```python
from build123d import *

# Parameters (mm, degrees)
BOSS_EXTRU_2_DEPTH      = 151.845
BOSS_EXTRU_2_DEPTH_BACK = 151.845
ESQUISSE1_R             = 7
ESQUISSE3_W             = 68
ESQUISSE3_H             = 30
ESQUISSE3_H_2           = 35
ESQUISSE4_R             = 5
BOSS_EXTRU_3_DEPTH      = 15
BOSS_EXTRU_4_START      = 15
ESQUISSE5_R             = 5
BOSS_EXTRU_4_DEPTH      = 15
BOSS_EXTRU_6_DEPTH      = 2.5
BOSS_EXTRU_6_DEPTH_BACK = 2.5
ENL_V_START             = -68
ESQUISSE11_R            = 35
ESQUISSE11_R_2          = 30
ENL_V_MAT_EXTRU_1_DEPTH = 68


with BuildPart() as part:
    # Esquisse1 → Boss.-Extru.2 (new, two sides: drawn at the far end of the back side and taken through both)
    with BuildSketch(Plane(origin=(0, 0, 0), x_dir=(0, 0, -1), z_dir=(1, 0, 0)).offset(-BOSS_EXTRU_2_DEPTH_BACK)):
        Circle(ESQUISSE1_R)
    extrude(amount=BOSS_EXTRU_2_DEPTH + BOSS_EXTRU_2_DEPTH_BACK)

    # Esquisse3 → Révolution2 (revolve)
    with BuildSketch(Plane.XY, mode=Mode.PRIVATE) as r_volution2_sk:
        with Locations((-86.5, 15)):
            Rectangle(ESQUISSE3_W, ESQUISSE3_H)
        with Locations((86.5, 17.5)):
            Rectangle(ESQUISSE3_W, ESQUISSE3_H_2)
    revolve(r_volution2_sk.sketch.rotate(Axis((-120.5, 0, 0), (1, 0, 0)), 270), axis=Axis((-120.5, 0, 0), (1, 0, 0)))

    # Esquisse4 → Boss.-Extru.3 (add)
    with BuildSketch(Plane.ZY.offset(151.845)):
        Circle(ESQUISSE4_R)
    extrude(amount=BOSS_EXTRU_3_DEPTH)

    # Esquisse5 → Boss.-Extru.4 (add)
    with BuildSketch(Plane(origin=(151.845, 0, 0), x_dir=(0, 0, -1), z_dir=(1, 0, 0)).offset(BOSS_EXTRU_4_START)):
        with Locations(Location((0, 0, 0), (0, 0, 180))):
            Circle(ESQUISSE5_R)
    extrude(amount=-BOSS_EXTRU_4_DEPTH)

    # Esquisse6 → Boss.-Extru.6 (add, two sides: drawn at the far end of the back side and taken through both)
    with BuildSketch(Plane(origin=(0, 0, 0), x_dir=(0, 0, -1), z_dir=(1, 0, 0)).offset(-BOSS_EXTRU_6_DEPTH_BACK)):
        Polygon((-0.495363477, 14), (-2.169953885, 6.655170932), (-2.610793017, 6.495072622), (-8.616105681, 11.046145282), (-9.378598341, 10.406337972), (-5.940243898, 3.703466513), (-6.175037056, 3.29745816), (-13.700746567, 2.923641509), (-13.873589621, 1.94339984), (-6.931134583, -0.98116596), (-6.850019438, -1.443108535), (-12.374762678, -6.566901532), (-11.87708094, -7.428911588), (-4.678977177, -5.206734889), (-4.319908407, -5.508463622), (-5.258596613, -12.984753276), (-4.323260899, -13.325187635), (-0.237581159, -6.99604961), (0.231428968, -6.996382273), (4.31801844, -13.326929566), (5.253354154, -12.986495207), (4.314874913, -5.51186988), (4.674371346, -5.210650816), (11.874077864, -7.433322313), (12.371759603, -6.571312256), (6.848246248, -1.448659888), (6.93001661, -0.986832845), (13.87401748, 1.938384149), (13.701174426, 2.918625818), (6.177140243, 3.292359253), (5.942923274, 3.698700268), (9.382043313, 10.403064212), (8.619550653, 11.042871522), (2.615574856, 6.492811995), (2.174963279, 6.653535506), (0.5, 14), align=None)
    extrude(amount=BOSS_EXTRU_6_DEPTH + BOSS_EXTRU_6_DEPTH_BACK)

    # Esquisse11 → Enlèv. mat.-Extru.1 (cut)
    with BuildSketch(Plane(origin=(120.5, 0, 0), x_dir=(0, 0, -1), z_dir=(1, 0, 0)).offset(ENL_V_START)):
        Circle(ESQUISSE11_R)
        with Locations(Location((0, 0, 0), (0, 0, 180))):
            Circle(ESQUISSE11_R_2, mode=Mode.SUBTRACT)
    extrude(amount=ENL_V_MAT_EXTRU_1_DEPTH, mode=Mode.SUBTRACT)


solid = part.part
```
Could you check a few things on this model? Use its own coordinates, in mm. A direction names the side the tool comes from. Round coordinates to 2 decimals unless told otherwise and drop trailing zeros. Loops run counter-clockwise (first coordinate to the right, second up) from the corner with the lowest first, then second, coordinate; pieces in that order, holes last. Notation, with made-up numbers: (60, 50.5) -> (88, 50.5) arc R30 cw to (88, 87.5) -> close; hole circle Ø10 at (-23.5, 76). An arc over 180 degrees is marked (long way). Put each result on its own line as item: value.
Q1. I want a section at B-B on z = 22. Write out the boundary of the cut face in (x, y).
Checks:
outline: (-120.5, -20.4) -> (-52.5, -20.4) -> (-52.5, 20.4) -> (-120.5, 20.4) -> close; (52.5, -20.4) -> (120.5, -20.4) -> (120.5, 20.4) -> (52.5, 20.4) -> close
Q2. Please list where these lines run through material, in increasing order: line 1 (X direction, y = -3.5, z = 9); line 2 (X direction, y = 22.5, z = -2); line 3 (Y direction, x = 131.5, z = -0.5). Write a range as from..to.
Checks:
line 1: -120.5..-52.5, -2.5..2.5, 52.5..120.5
line 2: -120.5..-52.5, 52.5..120.5
line 3: -6.98..6.98
Q3. Thinking about a two-plate mould opening in X: for faces 1 (the flat face through (-2.5, 7, 6)), 2 (the cylindrical face through (86.024, -25.296, 16.128)), 3 (the flat face through (-120.5, -6, 6)), which applies, pulls with the +X half, pulls with the -X half, needs draft (parallel to the pull), parting line crosses it, or undercut?
Checks:
face 1: undercut
face 2: needs draft
face 3: pulls with the -X half
Q4. Which directions (+Z, -Z, +X, -X, +Y, -Y) give clear straight access to the entire face, cutting with the end or side of a thin tool? Please do faces 4 (the flat face through (2.5, 7, -6)), 5 (the flat face through (2.5, 7, 6)), 6 (the flat face through (2.5, -5, -8)).
Checks:
face 4: -Z, +Y
face 5: +Z, +Y
face 6: -Z, -Y
Q5. I want a section at A-A on y = -24. Write out the boundary of the cut face in (x, z).
Checks:
outline: (-120.5, -18) -> (-52.5, -18) -> (-52.5, 18) -> (-120.5, 18) -> close; (52.5, -18) -> (120.5, -18) -> (120.5, 18) -> (52.5, 18) -> close
Q6. I want a section at C-C on x = 140.5. Write out the boundary of the cut face in (y, z).
Checks:
outline: circle Ø14 at (0, 0)
Q7. For pin 1 Ø2 at (x, z) = (-119.5, -9) entering from +Y; pin 2 Ø5.5 at (y, z) = (-10.5, 2.5) entering from -X; pin 3 Ø2 at (x, z) = (116, -20) entering from -Y; pin 4 Ø10 at (x, y) = (-15.5, 14.5) entering from +Z, each with a flat end and sliding along its axis, tell me the tip position at first contact or that it passes through.
Checks:
pin 1: y = 28.91
pin 2: x = -120.5
pin 3: y = -23.22
pin 4: through
